The model under review builds one solid part; all positions refer to its coordinate system, in mm. Face numbers are marked on the shaded views. A direction names the side the tool comes from. Round coordinates to 2 decimals unless told otherwise and drop trailing zeros. Write each loop counter-clockwise with the first axis right and the second up, starting at its lowest first coordinate (ties: lowest second). Pieces come first, ordered by that corner, then holes. Notation, with made-up numbers: (85, 73) - (128, 73) arc R8 cw to (128, 87) - close; hole circle Ø1 at (30.5, 49). An arc over 180 degrees is marked (long way). Return JSON: item names as keys, results as strings.
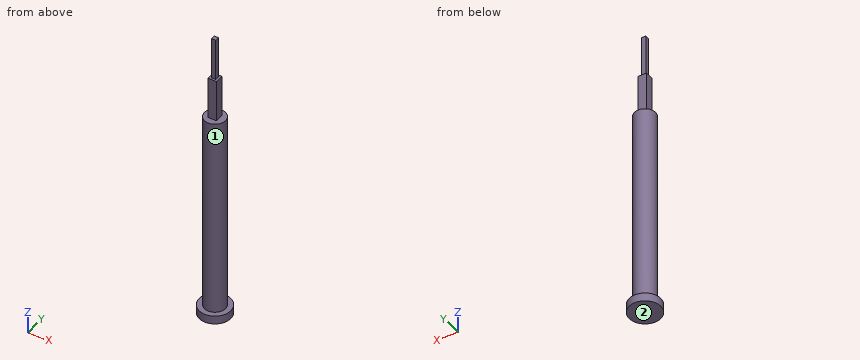
from build123d import *

# Parameters (mm, degrees)
F0_R     = 7.5
F1_DEPTH = 4
F2_R     = 5
F3_DEPTH = 100
F4_W     = 4
F4_H     = 4
F5_DEPTH = 20
F6_W     = 2
F6_H     = 2
F7_DEPTH = 20


with BuildPart() as f1:
    # F0 (on Top) → F1 (new body)
    with BuildSketch(Plane.XY):
        Circle(F0_R)
    extrude(amount=F1_DEPTH)

    # F2 (on Top) → F3 (join)
    with BuildSketch(Plane.XY):
        Circle(F2_R)
    extrude(amount=F3_DEPTH)

    # F4 (on face) → F5 (join)
    with BuildSketch(Plane.XY.offset(100)):
        Rectangle(F4_W, F4_H)
    extrude(amount=F5_DEPTH)

    # F6 (on face) → F7 (join)
    with BuildSketch(Plane.XY.offset(120)):
        Rectangle(F6_W, F6_H)
    extrude(amount=F7_DEPTH)


solid = f1.part
(1) Add section B-B (z = 32.5). Write out the cut boundary in (x, y), plus the area to 3 significant figures.
Filled in:
{"outline": "circle Ø10 at (0, 0)", "area": "78.5 mm2"}
(2) Clearance check with flat-ended pins moving along their axes: pin 1 Ø3 at (x, z) = (3, 91) entering from -Y; pin 2 Ø3 at (y, z) = (1, 106) entering from +X; pin 3 Ø2 at (x, z) = (-0.5, 127.5) entering from -Y; pin 4 Ø7.5 at (x, y) = (-2.5, 1.5) entering from +Z. State where each tip first meets the part, or that it passes through.
Filled in:
{"pin 1": "stops at y = -4.77", "pin 2": "stops at x = 2", "pin 3": "stops at y = -1", "pin 4": "stops at z = 140"}
(3) Add section C-C (z = 107). Write out the cut boundary in (x, y), plus the area to 3 significant figures.
Filled in:
{"outline": "(-2, -2) - (2, -2) - (2, 2) - (-2, 2) - close", "area": "16.0 mm2"}
(4) For the marked faces 1 and 2, list the 3-axis set-ups (+Z, -Z, +X, -X, +Y, -Y) from which the entire face can be reached by the end or side of a thin tool; tool diameter is ignored.
Filled in:
{"face 1": "+Z", "face 2": "-Z, +X, -X, +Y, -Y"}
(5) Wall thickness on line 1 (Z direction, x = 1.25, y = 5.75); line 2 (X direction, y = -0.25, z = 17); line 3 (Z direction, x = -3.25, y = -2.25): over which ranges is each line inside the solid? List them lowest first.
Filled in:
{"line 1": "z = 0 to 4", "line 2": "x = -4.99 to 4.99", "line 3": "z = 0 to 100"}
(6) Add section A-A (y = -3.5). Write out the cut boundary in (x, z), plus the area to 3 significant figures.
Filled in:
{"outline": "(-6.63, 0) - (6.63, 0) - (6.63, 4) - (3.57, 4) - (3.57, 100) - (-3.57, 100) - (-3.57, 4) - (-6.63, 4) - close", "area": "739 mm2"}
